Read the model definition and answer for the solid it produces. Units are mm, in the model's axes. Face numbers are marked on the shaded views. Coordinates: 2 decimals unless noted, no trailing zeros. Return JSON: item names as keys, results as strings. Group by question number.
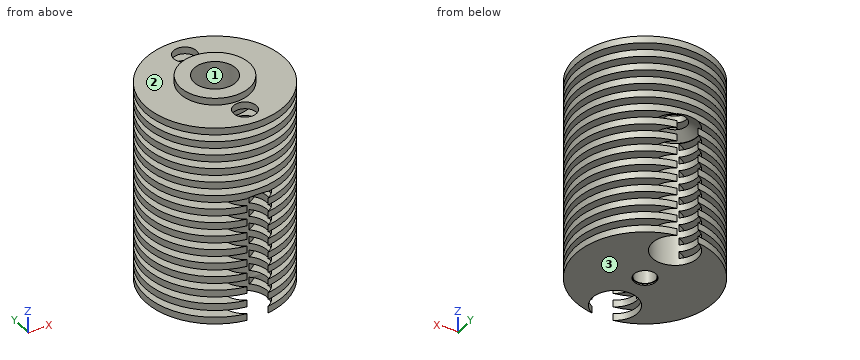
```python
from build123d import *

# Parameters (mm, degrees)
LINEARPATTERN_COUNT = 15
LINEARPATTERN_PITCH = 2
SKETCH011_R         = 1.65
HOLE007_DEPTH       = 29.001
SKETCH014_R         = 3.25
HOLE008_DEPTH       = 18.047203
HOLE008_TIPS_R      = 3.25


with BuildPart() as part:
    # Sketch008 → Revolution (revolve)
    with BuildSketch(Plane.XZ):
        Polygon((0, 14.5), (10, 14.5), (10, 15.5), (5, 15.5), (5, 16.5), (0, 16.5), align=None)
    revolution = revolve(axis=Axis((0, 0, 0), (0, 0, 1)))

    # LinearPattern: Revolution ×15
    with Locations(*[(0, 0, i * LINEARPATTERN_PITCH) for i in range(1, LINEARPATTERN_COUNT)]):
        add(revolution)

    # Sketch009 → Groove (revolve, cut)
    with BuildSketch(Plane.XZ):
        Polygon((1.6, 14.5), (1.6, 14.7), (1.5, 14.7), (1.5, 34.5), (3, 34.5), (3, 44.5), (0, 44.5), (0, 14.5), align=None)
    revolve(axis=Axis((0, 0, 0), (0, 0, 1)), mode=Mode.SUBTRACT)

    # Sketch011 → Hole007 (cut, through all)
    with BuildSketch(Plane(origin=(0, 0, 43.5), x_dir=(-1, 0, 0), z_dir=(0, 0, 1))):
        with Locations((0, 7)):
            Circle(SKETCH011_R)
        with Locations((0, -7)):
            Circle(SKETCH011_R)
    extrude(amount=-HOLE007_DEPTH, mode=Mode.SUBTRACT)

    # Sketch014 (on Face97 of Hole007) → Hole008 (cut)
    with BuildSketch(Plane(origin=(0, 0, 14.5), x_dir=(1, 0, 0), z_dir=(0, 0, -1))):
        with Locations((0, 7)):
            Circle(SKETCH014_R)
        with Locations((0, -7)):
            Circle(SKETCH014_R)
    extrude(amount=-HOLE008_DEPTH, mode=Mode.SUBTRACT)

    # Hole008 tips → Hole008 tip 1 section 0
    with BuildSketch(Plane(origin=(0, 0, 32.547203), x_dir=(1, 0, 0), z_dir=(0, 0, -1)), mode=Mode.PRIVATE) as hole008_tip_1_s0:
        with Locations((0, 7)):
            Circle(HOLE008_TIPS_R)
    loft([hole008_tip_1_s0.sketch, Vertex(0, -7, 34.5)], mode=Mode.SUBTRACT)

    # Hole008 tips → Hole008 tip 2 section 0
    with BuildSketch(Plane(origin=(0, 0, 32.547203), x_dir=(1, 0, 0), z_dir=(0, 0, -1)), mode=Mode.PRIVATE) as hole008_tip_2_s0:
        with Locations((0, -7)):
            Circle(HOLE008_TIPS_R)
    loft([hole008_tip_2_s0.sketch, Vertex(0, 7, 34.5)], mode=Mode.SUBTRACT)


solid = part.part
```
1. Given pin 1 (1.5 mm diameter, centred on x = 6.5, z = 19, fed in from +Y); pin 2 (4 mm diameter, centred on x = -4.5, z = 19.5, fed in from -Y); pin 3 (2.5 mm diameter, centred on x = -6.5, y = -5, fed in from +Z); pin 4 (2.5 mm diameter, centred on x = 0, y = -7, fed in from -Z), each flat-ended and moving along its own axis, determine where each tip first touches the part or whether it passes through.
2. For a pull along Z with two mould halves and no side action, classify the marked faces 1, 2 and 3 as released by +Z, released by -Z, zero draft, split by the parting line, or undercut.
3. Find section A-A on y = -7. Give the number of separate pieces and of enclosed holes in the cut face, and give its area (3 significant figures).
4. Straight lines are drawn through the part: L1, parallel to Y at x = 0, z = 40.75; L2, parallel to Y at x = 0, z = 20.5; L3, parallel to Y at x = 2.75, z = 25. For each, find the intervals that lie inside material, in ascending order.
Result:
{
 "1": {"pin 1": "y = 8.18", "pin 2": "y = -9.68", "pin 3": "z = 43.5", "pin 4": "through"},
 "2": {"face 1": "zero draft", "face 2": "released by +Z", "face 3": "released by -Z"},
 "3": {"separate pieces": "30", "enclosed holes": "0", "area": "134 mm^2"},
 "4": {"L1": "-10 to -8.65, -5.35 to -3, 3 to 5.35, 8.65 to 10", "L2": "-3.75 to -1.5, 1.5 to 3.75", "L3": "-9.61 to -8.73, -5.27 to 5.27, 8.73 to 9.61"}
}
